The listing builds one solid part. Answer for the finished solid, in the listing's coordinates (mm). Face numbers are marked on the shaded views. A direction names the side the tool comes from. Coordinates: 2 decimals unless noted, no trailing zeros. Loops run counter-clockwise (first coordinate to the right, second up) from the corner with the lowest first, then second, coordinate; pieces in that order, holes last. Notation, with made-up numbers: (54.25, -12.75) - (86.25, -12.75) arc R16 cw to (86.25, 5.25) - close; hole circle Ø11 at (55, 6.5). An arc over 180 degrees is marked (long way). Write each question's results on one line, items separated by ' | '. Start each with the question number.
(1) Find section A-A on y = 0. State how many separate pieces and enclosed holes the cut face has, then the cut area to 3 significant figures.
(2) Determine the mould class of the marked faces 3, 4 and 5 for opening direction Y: released by +Y, released by -Y, zero draft, split by the parting line, or undercut.
(3) Given pin 1 Ø1.5 at (x, y) = (-12, 9) entering from +Z; pin 2 Ø8 at (x, y) = (-2.5, 13.5) entering from -Z; pin 3 Ø8 at (x, y) = (10.5, -12.5) entering from -Z, each flat-ended and moving along its own axis, determine where each tip first touches the part or whether it passes through.
(4) Consider line 1 (X direction, y = 28, z = -10.5); line 2 (Z direction, x = 18.5, y = 23); line 3 (Z direction, x = -10, y = -9). Determine where each line is inside the solid, lowest interval first. Write a range as from..to.
(5) Find section C-C on x = 10.5. Determine the outline of the cut face in (y, z), then the cut area to 3 significant figures.
(6) Find section D-D on x = 16.5. Determine the outline of the cut face in (y, z).
(7) For the marked faces 1 and 2, determine the directions among +Z, -Z, +X, -X, +Y, -Y from which every point of the face is accessible in a straight line to the end or side of a thin tool.
(8) Find section B-B on x = -5. Determine the outline of the cut face in (y, z), then the cut area to 3 significant figures.
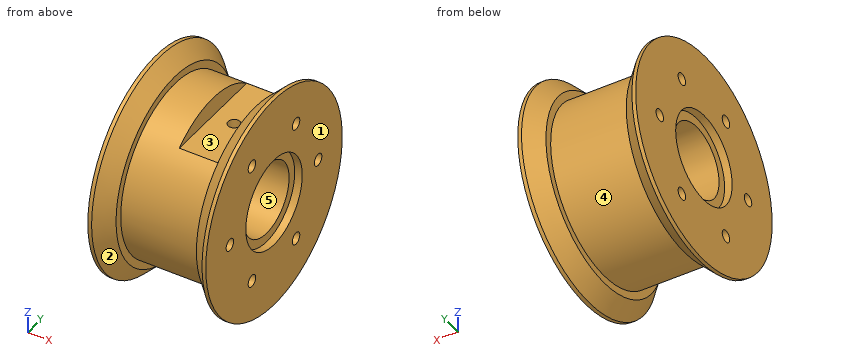
from build123d import *

# Parameters (mm, degrees)
SKETCH4_R                  = 15.24
CUT_EXTRUDE1_DEPTH         = 2.54
CIRPATTERN1_COUNT          = 6
CUT_EXTRUDE3_DEPTH         = 56.771511733
CUT_EXTRUDE3_DEPTH_BACK    = 56.771511733
SKETCH9_W                  = 14.2875
SKETCH9_H                  = 6.35
F_10_32_TAPPED_HOLE2_D     = 4.0386
F_10_32_TAPPED_HOLE2_DEPTH = 11.938
F_10_32_TAPPED_HOLE2_TIP   = 1.213317848
CHAMFER1_SIZE              = 5.08


with BuildPart() as part:
    # Sketch3 → Revolve1 (revolve)
    with BuildSketch(Plane.XY, mode=Mode.PRIVATE) as revolve1_sk:
        Polygon((-19.939, 12.192), (19.939, 12.192), (19.939, 36.83), (13.589, 36.83), (13.589, 29.21), (-13.589, 29.21), (-13.589, 36.83), (-19.939, 36.83), align=None)
    revolve(revolve1_sk.sketch.rotate(Axis((-36.327412464, 0, 0), (1, 0, 0)), 180), axis=Axis((-36.327412464, 0, 0), (1, 0, 0)))

    # Sketch4 → Cut-Extrude1 (cut)
    with BuildSketch(Plane(origin=(19.939, 0, 0), x_dir=(0, 0, -1), z_dir=(1, 0, 0))):
        with Locations(Location((0, 0, 0), (0, 0, 90))):
            Circle(SKETCH4_R)
    cut_extrude1 = extrude(amount=-CUT_EXTRUDE1_DEPTH, mode=Mode.SUBTRACT)

    # Mirror1: Cut-Extrude1 across plane
    add(cut_extrude1.mirror(Plane(origin=(0, 0, 0), x_dir=(0, 0, 1), z_dir=(1, 0, 0))), mode=Mode.SUBTRACT)

    # Sketch7 → #10-32 Tapped Hole1 (revolve, cut)
    with BuildSketch(Plane(origin=(19.939, -23.8125, 0), x_dir=(0, 0, -1), z_dir=(0, 1, 0))):
        Polygon((0, 0), (0, 13.151317848), (2.0193, 11.938), (2.0193, 0), align=None)
    f_10_32_tapped_hole1 = revolve(axis=Axis((26.289, -23.8125, 0), (-1, 0, 0)), mode=Mode.SUBTRACT)

    # CirPattern1: #10-32 Tapped Hole1 ×6 about axis
    cirpattern1_axis = Axis((0, 0, 0), (1, 0, 0))
    for i in range(1, CIRPATTERN1_COUNT):
        add(f_10_32_tapped_hole1.rotate(cirpattern1_axis, i * 360 / CIRPATTERN1_COUNT), mode=Mode.SUBTRACT)

    # Mirror2: #10-32 Tapped Hole1 across plane
    add(f_10_32_tapped_hole1.mirror(Plane(origin=(0, 0, 0), x_dir=(0, 0, 1), z_dir=(1, 0, 0))), mode=Mode.SUBTRACT)

    # Mirror2 copy 1 sketch → Mirror2 copy 1 (revolve, cut)
    with BuildSketch(Plane(origin=(-19.939, -11.90625, -20.622229928), x_dir=(0, 0.8660254037844386, -0.5000000000000001), z_dir=(0, 0.5000000000000001, 0.8660254037844386))):
        Polygon((0, 0), (0, -13.151317848), (2.0193, -11.938), (2.0193, 0), align=None)
    revolve(axis=Axis((-26.289, -11.90625, -20.622229928), (-1, 0, 0)), mode=Mode.SUBTRACT)

    # Mirror2 copy 2 sketch → Mirror2 copy 2 (revolve, cut)
    with BuildSketch(Plane(origin=(-19.939, 11.90625, -20.622229928), x_dir=(0, 0.8660254037844387, 0.4999999999999998), z_dir=(0, -0.4999999999999998, 0.8660254037844387))):
        Polygon((0, 0), (0, -13.151317848), (2.0193, -11.938), (2.0193, 0), align=None)
    revolve(axis=Axis((-26.289, 11.90625, -20.622229928), (-1, 0, 0)), mode=Mode.SUBTRACT)

    # Mirror2 copy 3 sketch → Mirror2 copy 3 (revolve, cut)
    with BuildSketch(Plane(origin=(-19.939, 23.8125, 0), x_dir=(0, 0, 1), z_dir=(0, -1, 0))):
        Polygon((0, 0), (0, -13.151317848), (2.0193, -11.938), (2.0193, 0), align=None)
    revolve(axis=Axis((-26.289, 23.8125, 0), (-1, 0, 0)), mode=Mode.SUBTRACT)

    # Mirror2 copy 4 sketch → Mirror2 copy 4 (revolve, cut)
    with BuildSketch(Plane(origin=(-19.939, 11.90625, 20.622229928), x_dir=(0, -0.8660254037844384, 0.5000000000000004), z_dir=(0, -0.5000000000000004, -0.8660254037844384))):
        Polygon((0, 0), (0, -13.151317848), (2.0193, -11.938), (2.0193, 0), align=None)
    revolve(axis=Axis((-26.289, 11.90625, 20.622229928), (-1, 0, 0)), mode=Mode.SUBTRACT)

    # Mirror2 copy 5 sketch → Mirror2 copy 5 (revolve, cut)
    with BuildSketch(Plane(origin=(-19.939, -11.90625, 20.622229928), x_dir=(0, -0.8660254037844386, -0.5000000000000001), z_dir=(0, 0.5000000000000001, -0.8660254037844386))):
        Polygon((0, 0), (0, -13.151317848), (2.0193, -11.938), (2.0193, 0), align=None)
    revolve(axis=Axis((-26.289, -11.90625, 20.622229928), (-1, 0, 0)), mode=Mode.SUBTRACT)

    # Sketch9 → Cut-Extrude3 (cut, two sides: drawn at the far end of the back side and taken through both)
    with BuildSketch(Plane(origin=(0, 0, 0), x_dir=(1, 0, 0), z_dir=(0, 1, 0)).offset(-CUT_EXTRUDE3_DEPTH_BACK)):
        with Locations((6.44525, -26.035)):
            Rectangle(SKETCH9_W, SKETCH9_H)
    extrude(amount=CUT_EXTRUDE3_DEPTH + CUT_EXTRUDE3_DEPTH_BACK, mode=Mode.SUBTRACT)

    # #10-32 Tapped Hole2
    with Locations(Plane.XY.offset(22.86)):
        with Locations((6.44525, 0)):
            Hole(F_10_32_TAPPED_HOLE2_D / 2, depth=F_10_32_TAPPED_HOLE2_DEPTH)
            with Locations((0, 0, -(F_10_32_TAPPED_HOLE2_DEPTH + F_10_32_TAPPED_HOLE2_TIP / 2))):  # 118° drill point
                Cone(0, F_10_32_TAPPED_HOLE2_D / 2, F_10_32_TAPPED_HOLE2_TIP, mode=Mode.SUBTRACT)

    # Chamfer1
    chamfer1_edges = [part.edges().sort_by_distance(p)[0] for p in [
        (-13.589, 36.83, 0),
        (13.589, 36.83, 0),
    ]]
    chamfer(chamfer1_edges, length=CHAMFER1_SIZE)


solid = part.part
Values:
1) separate pieces: 3 | enclosed holes: 0 | area: 1,330 mm²
2) face 3: zero draft | face 4: split by the parting line | face 5: undercut
3) pin 1: stops at z = 28.02 | pin 2: stops at z = -27.62 | pin 3: stops at z = -30.45
4) line 1: x = -19.94..-13.59, 13.59..19.94 | line 2: z = -28.55..-1.85, 1.85..28.55 | line 3: z = -27.79..-8.22, 8.22..27.79
5) outline: (-18.18, 22.86) arc R29.21 ccw (long way) to (18.18, 22.86) - close; hole circle Ø4.04 at (-23.81, 0); hole circle Ø4.04 at (-11.91, -20.62); hole circle Ø4.04 at (-11.91, 20.62); hole circle Ø24.38 at (0, 0); hole circle Ø4.04 at (11.91, -20.62); hole circle Ø4.04 at (11.91, 20.62); hole circle Ø4.04 at (23.81, 0) | area: 1,980 mm²
6) outline: circle Ø69.32 at (0, 0); hole circle Ø4.04 at (-23.81, 0); hole circle Ø4.04 at (-11.91, -20.62); hole circle Ø4.04 at (-11.91, 20.62); hole circle Ø24.38 at (0, 0); hole circle Ø4.04 at (11.91, -20.62); hole circle Ø4.04 at (11.91, 20.62); hole circle Ø4.04 at (23.81, 0)
7) face 1: +Z, -Z, +X, +Y, -Y | face 2: none
8) outline: circle Ø58.42 at (0, 0); hole circle Ø24.38 at (0, 0) | area: 2,210 mm²
